Source: CAD feature listing. Evaluate the final solid. Frame: model axes, mm. Coordinates: 2 decimals unless noted, no trailing zeros. Loops run counter-clockwise (first coordinate to the right, second up) from the corner with the lowest first, then second, coordinate; pieces in that order, holes last.
Autodesk Inventor part; units mm, degrees
ref_plane "YZ Plane" through (0, 0, 0) normal (1, 0, 0) x (0, 1, 0)
ref_plane "XZ Plane" through (0, 0, 0) normal (0, 1, 0) x (-1, 0, 0)
ref_plane "XY Plane" through (0, 0, 0) normal (0, 0, 1) x (1, 0, 0)
sketch "Sketch1" plane through (0, 0, 0) normal (0, 1, 0) x (-1, 0, 0)
  line L0 (-47.5, 47.5) -> (47.5, 47.5)
  line L1 (47.5, 47.5) -> (47.5, -47.5)
  line L2 (47.5, -47.5) -> (-47.5, -47.5)
  line L3 (-47.5, -47.5) -> (-47.5, 47.5)
  line L4 (-47.5, 47.5) -> (47.5, -47.5) construction
  line L5 (47.5, 47.5) -> (-47.5, -47.5) construction
  point P0 (0, 0)
  dimension "d0" = 95
  dimension "d1" = 95
extrude "Extrusion1" add sketch "Sketch1" along normal blind 1.6
sketch "Sketch4" plane through (0, 1.6, 0) normal (0, 1, 0) x (1, 0, 0)
  line L0 (-47.5, 47.5) -> (-47.5, -47.5)
  line L1 (-47.5, -47.5) -> (-36.5, -47.5)
  line L2 (-36.5, -47.5) -> (-36.5, -27.5)
  line L3 (-36.5, -27.5) -> (-47.5, -27.5)
  line L4 (-47.5, -27.5) -> (-47.5, -47.5)
  line L5 (-47.5, -47.5) -> (47.5, -47.5)
  line L6 (47.5, -47.5) -> (36.5, -47.5)
  line L7 (36.5, -47.5) -> (36.5, -27.5)
  line L8 (36.5, -27.5) -> (47.5, -27.5)
  line L9 (47.5, -27.5) -> (47.5, -47.5)
  line L10 (-47.5, 47.5) -> (-36.5, 47.5)
  line L11 (-36.5, 47.5) -> (-36.5, 27.5)
  line L12 (-36.5, 27.5) -> (-47.5, 27.5)
  line L13 (-47.5, 27.5) -> (-47.5, 47.5)
  line L14 (47.5, 47.5) -> (-47.5, 47.5)
  line L15 (47.5, 47.5) -> (36.5, 47.5)
  line L16 (36.5, 47.5) -> (36.5, 27.5)
  line L17 (36.5, 27.5) -> (47.5, 27.5)
  line L18 (47.5, 27.5) -> (47.5, 47.5)
  point P0 (0, 0)
  point P1 (-47.5, -27.5)
  point P2 (-47.5, 27.5)
  dimension "d18" = 11
  dimension "d19" = 20
  dimension "d21" = 20
  dimension "d22" = 11
  dimension "d23" = 11
  dimension "d24" = 20
  dimension "d25" = 11
  dimension "d26" = 20
extrude "Extrusion2" cut sketch "Sketch4" against normal blind 1.6
fillet "Fillet1" radius 4 4 edges at (36.5, 0.8, -27.5) (36.5, 0.8, 27.5) (-36.5, 0.8, 27.5) (-36.5, 0.8, -27.5)
fillet "Fillet2" radius 3 8 edges at (36.5, 0.8, 47.5) (-36.5, 0.8, 47.5) (-36.5, 0.8, -47.5) (36.5, 0.8, -47.5) (-47.5, 0.8, -27.5) (47.5, 0.8, -27.5) (47.5, 0.8, 27.5) (-47.5, 0.8, 27.5)
sketch "Sketch6" plane through (0, 1.6, 0) normal (0, 1, 0) x (1, 0, 0)
  line L0 (31.5, 29) -> (-25.5, 29) construction
  line L1 (-25.5, 29) -> (-25.5, -29) construction
  line L2 (-25.5, -29) -> (31.5, -29) construction
  line L3 (31.5, -29) -> (31.5, 29) construction
  line L4 (31.5, 29) -> (-25.5, -29) construction
  line L5 (-25.5, 29) -> (31.5, -29) construction
  line L6 (-66.5, 0) -> (66.5, 0) construction
  line L7 (0, 66.5) -> (0, -66.5) construction
  point P0 (3, 0)
  dimension "d31" = 57
  dimension "d32" = 58
  dimension "d41" = 3
hole "Hole2" at (-25.5, 1.6, 29) at (-25.5, 1.6, -29) at (31.5, 1.6, -29) at (31.5, 1.6, 29) direction (0, -1, 0) diameter 4.2 end through all
sketch "Sketch7" plane through (0, 1.6, 0) normal (0, 1, 0) x (1, 0, 0)
  line L0 (-47.5, 24.5) -> (-47.5, -24.5)
  line L1 (-36.5, -31.5) -> (-47.5, -31.5)
  line L2 (-47.5, -31.5) -> (-47.5, -9.5)
  line L3 (-47.5, -9.5) -> (-36.5, -9.5)
  line L4 (-36.5, -9.5) -> (-36.5, -31.5)
  point P0 (0, 0)
  dimension "d45" = 22
extrude "Extrusion3" cut sketch "Sketch7" against normal blind 10
fillet "Fillet3" radius 3 1 edges at (-47.5, 0.8, 9.5)
fillet "Fillet4" radius 4 1 edges at (-36.5, 0.8, 9.5)
equation "\"d19\" = d21"
equation "\"d22\" = d18"
equation "\"d23\" = d18"
equation "\"d24\" = d19"
equation "\"d25\" = d18"
equation "\"d26\" = d21"
properties part number "pcbIO"
Q1. Section A-A, the plane y = 1.05. Return the cut outline in (x, z).
Q2. Contact query for flat-ended pins moving along their axis: pin 1 Ø2.5 at (x, z) = (-25.5, 29) entering from +Y; pin 2 Ø0.5 at (y, z) = (1, 28.5) entering from -X; pin 3 Ø0.5 at (x, y) = (42, 0.5) entering from +Z; pin 4 Ø0.5 at (y, z) = (1, 39.5) entering from +X. Output: stop coordinate, or through.
Q3. Line query: line 1 along Z through (x, y) = (31.5, 0.55); line 2 along X through (y, z) = (0.9, -29); line 3 along X through (y, z) = (1.05, 29). Output: solid intervals per line, ascending.
Q4. Draft query along X for faces 1 (the cylindrical face through (-25.59, 0.79, 26.9)), 2 (the flat face through (1, 0, 1)), 3 (the cylindrical face through (-46.6, 0.79, 8.64)). Return one class per face: +X half, -X half, draft (parallel to the pull), parting line (faces both ways), or undercut.
Q5. Section C-C, the plane z = 29. Return the cut outline in (x, y).
Q6. Section B-B, the plane x = -25.5. Return the cut outline in (y, z), plus the area to 3 significant figures.
Derived:
1. outline: (-47.5, -24.5) arc R3 ccw to (-44.5, -27.5) - (-40.5, -27.5) arc R4 cw to (-36.5, -31.5) - (-36.5, -44.5) arc R3 ccw to (-33.5, -47.5) - (33.5, -47.5) arc R3 ccw to (36.5, -44.5) - (36.5, -31.5) arc R4 cw to (40.5, -27.5) - (44.5, -27.5) arc R3 ccw to (47.5, -24.5) - (47.5, 24.5) arc R3 ccw to (44.5, 27.5) - (40.5, 27.5) arc R4 cw to (36.5, 31.5) - (36.5, 44.5) arc R3 ccw to (33.5, 47.5) - (-33.5, 47.5) arc R3 ccw to (-36.5, 44.5) - (-36.5, 13.5) arc R4 cw to (-40.5, 9.5) - (-44.5, 9.5) arc R3 ccw to (-47.5, 6.5) - close; hole circle Ø4.2 at (-25.5, -29); hole circle Ø4.2 at (-25.5, 29); hole circle Ø4.2 at (31.5, -29); hole circle Ø4.2 at (31.5, 29)
2. pin 1: passes through
2. pin 2: stops at x = -36.5
2. pin 3: stops at z = 27.5
2. pin 4: stops at x = 36.5
3. line 1: z = -47.5 to -31.1, -26.9 to 26.9, 31.1 to 47.5
3. line 2: x = -37.38 to -27.6, -23.4 to 29.4, 33.6 to 37.38
3. line 3: x = -36.5 to -27.6, -23.4 to 29.4, 33.6 to 37.38
4. face 1: undercut
4. face 2: draft
4. face 3: -X half
5. outline: (-36.5, 0) - (-27.6, 0) - (-27.6, 1.6) - (-36.5, 1.6) - close; (-23.4, 0) - (29.4, 0) - (29.4, 1.6) - (-23.4, 1.6) - close; (33.6, 0) - (37.38, 0) - (37.38, 1.6) - (33.6, 1.6) - close
6. outline: (0, -47.5) - (1.6, -47.5) - (1.6, -31.1) - (0, -31.1) - close; (0, -26.9) - (1.6, -26.9) - (1.6, 26.9) - (0, 26.9) - close; (0, 31.1) - (1.6, 31.1) - (1.6, 47.5) - (0, 47.5) - close
6. area: 139 mm2
